Autodesk Inventor part; units mm, degrees
ref_plane "YZ Plane" through (0, 0, 0) normal (1, 0, 0) x (0, 1, 0)
ref_plane "XZ Plane" through (0, 0, 0) normal (0, 1, 0) x (-1, 0, 0)
ref_plane "XY Plane" through (0, 0, 0) normal (0, 0, 1) x (1, 0, 0)
sketch "Sketch1" plane through (0, 0, 0) normal (0, 1, 0) x (-1, 0, 0)
  line L0 (0, 0) -> (31, 0)
  line L1 (31, 0) -> (31, -32)
  line L2 (31, -32) -> (0, -32)
  line L3 (0, -32) -> (0, 0)
  dimension "d0" = 31
  dimension "d1" = 32
extrude "Extrusion1" add sketch "Sketch1" along normal blind 3
sketch "Sketch2" plane through (-31, 0, -32) normal (-1, 0, 0) x (0, 0, 1)
  line L0 (32, 3) -> (0, 3)
  line L1 (0, 3) -> (0, -15)
  line L2 (0, -15) -> (32, -15)
  line L3 (32, -15) -> (32, 3)
  point P0 (32, 0)
  dimension "d4" = 32
  dimension "d5" = 18
extrude "Extrusion2" add sketch "Sketch2" along normal blind 3
sketch "Sketch3" plane through (0, 0, 0) normal (1, 0, 0) x (0, 0, -1)
  line L0 (0, 3) -> (32, 3)
  line L1 (32, 3) -> (32, -15)
  line L2 (32, -15) -> (0, -15)
  line L3 (0, -15) -> (0, 3)
  point P0 (0, 0)
  dimension "d8" = 32
  dimension "d9" = 18
extrude "Extrusion3" add sketch "Sketch3" along normal blind 3
sketch "Sketch4" plane through (3, 0, 0) normal (1, 0, 0) x (0, 0, -1)
  line L0 (0, 3) -> (0, -15)
  line L1 (0, -15) -> (32, -15)
  line L2 (32, -15) -> (32, -12)
  line L3 (32, -12) -> (0, -12)
  line L4 (0, -12) -> (0, -15)
  point P0 (0, 0)
  dimension "d12" = 32
  dimension "d13" = 3
extrude "Extrusion4" add sketch "Sketch4" along normal blind 6
sketch "Sketch5" plane through (-34, 0, -32) normal (-1, 0, 0) x (0, 0, 1)
  line L0 (0, -15) -> (32, -15)
  line L1 (0, -15) -> (32, -15)
  line L2 (32, -15) -> (32, -12)
  line L3 (32, -12) -> (0, -12)
  line L4 (0, -12) -> (0, -15)
  point P0 (32, 0)
  dimension "d16" = 32
  dimension "d17" = 3
extrude "Extrusion5" add sketch "Sketch5" along normal blind 6
sketch "Sketch6" plane through (-34, -12, 0) normal (0, 1, 0) x (1, 0, 0)
  circle A0 centre (40, 28.97) radius 2
  circle A1 centre (40, 3.5) radius 2
  circle A2 centre (-3, 28.97) radius 2
  circle A3 centre (-3, 3.5) radius 2
  line L0 (37, 0) -> (43, 0)
  line L1 (0, 0) -> (-6, 0)
  line L2 (43, 32) -> (43, 0)
  line L3 (-6, 0) -> (-6, 32)
  point P0 (34, 0)
  dimension "d20" = 4
  dimension "d21" = 4
  dimension "d22" = 4
  dimension "d23" = 4
  dimension "d24" = 25.47
  dimension "d25" = 25.47
  dimension "d26" = 3.5
  dimension "d27" = 3.5
  dimension "d28" = 3
  dimension "d29" = 3
  dimension "d30" = 3
extrude "Extrusion6" cut sketch "Sketch6" against normal blind 6
sketch "Sketch7" plane through (0, 0, 0) normal (0, -1, 0) x (1, 0, 0)
  line L0 (0, -32) -> (9, -32)
  line L1 (-31, -32) -> (-31, 0)
  line L2 (0, -32) -> (-31, -32)
  line L3 (-31, -32) -> (-31, -29)
  line L4 (-31, -29) -> (0, -29)
  line L5 (0, -29) -> (0, -32)
  point P0 (0, 0)
  dimension "d33" = 3
extrude "Extrusion7" add sketch "Sketch7" along normal blind 11.7
properties part number "AprieteEthernet"
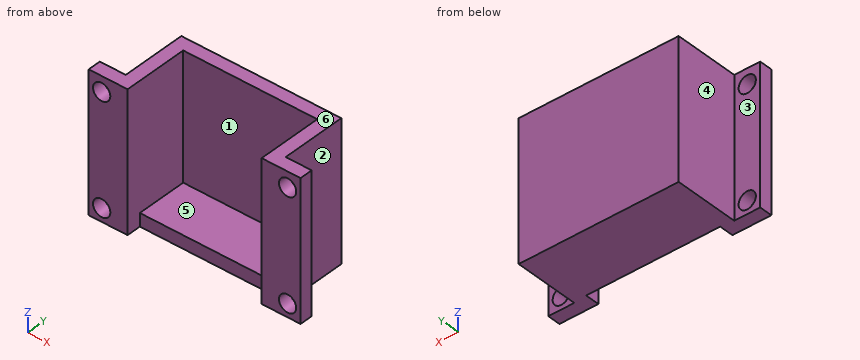
CAD build for the part. Positions are in the model's coordinates, mm. Face numbers are marked on the shaded views. A direction names the side the tool comes from. Round coordinates to 2 decimals unless told otherwise and drop trailing zeros. Order: outer loops, then holes, each group sorted by start corner. A loop starts at its lowest first (then second) coordinate and runs counter-clockwise, first axis right, second up. Notation, with made-up numbers: (36, -38.75) -> (87, -38.75) arc R13 cw to (87, -25.75) -> close; hole circle Ø11 at (23.25, -6.5). An arc over 180 degrees is marked (long way). Write item = value, one per line. Start each with the question number.
(1) Cut at D-D, the plane y = -3.75. List the corners of the cut face in (x, z), then the cut area to 3 significant figures.
(2) Pin check, flat tips, straight feed: P1, Ø1.5, axis at x = -28.5, y = -7, coming from the +Z side; P2, Ø4.5, axis at x = -37, z = -28.97, coming from the +Y side; P3, Ø1, axis at x = -13, z = -25, coming from the -Y side. Stop position of each tip, or through.
(3) Cut at B-B, the plane z = -3.5. List the corners of the cut face in (x, y).
(4) Pull direction X, two halves, no side cores. Call the marked faces 4, 5 and 6: released by +X, released by -X, zero draft, split by the parting line, or undercut.
(5) Probe line 1 (X direction, y = -14.15, z = -3.5); line 2 (Z direction, x = -37, y = -13.9); line 3 (X direction, y = -11.25, z = -27.5). List the from-to ranges inside material, lowest first. Write a range as [from, to].
(6) Which spindle directions (+Z, -Z, +X, -X, +Y, -Y) get a long thin tool onto all of the face, cutting with end or side? Do the marked faces 1, 2 and 3. Say none if no direction does.
(7) Cut at A-A, the plane y = -13. List the corners of the cut face in (x, z), then the cut area to 3 significant figures.
(8) Cut at C-C, the plane x = -37. List the corners of the cut face in (y, z), then the cut area to 3 significant figures.
Model answer:
q1.outline = (-34, -32) -> (3, -32) -> (3, 0) -> (0, 0) -> (0, -29) -> (-31, -29) -> (-31, 0) -> (-34, 0) -> close
q1.area = 285 mm2
q2.P1 = -29
q2.P2 = -12
q2.P3 = 0
q3.outline = (-40, -15) -> (-39, -15) -> (-39, -12) -> (-40, -12) -> close; (-35, -15) -> (-31, -15) -> (-31, 0) -> (0, 0) -> (0, -15) -> (4, -15) -> (4, -12) -> (3, -12) -> (3, 3) -> (-34, 3) -> (-34, -12) -> (-35, -12) -> close; (8, -15) -> (9, -15) -> (9, -12) -> (8, -12) -> close
q4.face_4 = released by -X
q4.face_5 = undercut
q4.face_6 = zero draft
q5.line_1 = [-40, -39], [-35, -31], [0, 4], [8, 9]
q5.line_2 = [-32, -30.97], [-26.97, -5.5], [-1.5, 0]
q5.line_3 = [-34, -31], [0, 3]
q6.face_1 = +Z, -Y
q6.face_2 = +Z, -Z, +X, +Y
q6.face_3 = +Z, -Z, -X, +Y
q7.outline = (-40, -32) -> (-31, -32) -> (-31, 0) -> (-40, 0) -> close; (0, -32) -> (9, -32) -> (9, 0) -> (0, 0) -> close; hole circle Ø4 at (-37, -28.97); hole circle Ø4 at (-37, -3.5); hole circle Ø4 at (6, -28.97); hole circle Ø4 at (6, -3.5)
q7.area = 526 mm2
q8.outline = (-15, -32) -> (-12, -32) -> (-12, -30.97) -> (-15, -30.97) -> close; (-15, -26.97) -> (-12, -26.97) -> (-12, -5.5) -> (-15, -5.5) -> close; (-15, -1.5) -> (-12, -1.5) -> (-12, 0) -> (-15, 0) -> close
q8.area = 72.0 mm2
